Could you check a few things on this model? Use its own coordinates, in mm. A direction names the side the tool comes from. Give positions to 0.01 mm unless a question says otherwise; leave off trailing zeros. Loops run counter-clockwise (first coordinate to the right, second up) from the corner with the lowest first, then second, coordinate; pieces in that order, holes last. Notation, with made-up numbers: (88.25, 35.5) - (96.25, 35.5) arc R26 cw to (96.25, 59.5) - close; hole circle Ø1 at (37, 33). An arc over 180 degrees is marked (long way). Write each question's results on one line, items separated by ' | '. Start each with the question number.
(1) Suppose I cut it at B-B (y = 7.5). Please give me the cut outline in (x, z).
(2) Suppose I cut it at D-D (y = 4.75). Please give me the cut outline in (x, z), and give its area (3 significant figures).
(3) Suppose I cut it at C-C (x = -9.3). Please give me the cut outline in (y, z).
(4) For pin 1 (5 mm diameter, centred on x = -9.5, z = -17.5, fed in from +Y); pin 2 (8 mm diameter, centred on x = -13, z = -16.5, fed in from -Y); pin 3 (10 mm diameter, centred on x = -16.5, y = 16, fed in from -Z); pin 4 (3 mm diameter, centred on x = -4.5, z = -4.9, fed in from -Y), each with a flat end and sliding along its axis, tell me the tip position at first contact or that it passes through.
(5) Suppose I cut it at A-A (z = -4.9). Please give me the cut outline in (x, y).
(6) I need wall thicknesses on line 1 (X direction, y = 5.25, z = -30.1); line 2 (Z direction, x = -4.5, y = 3.75); line 3 (Z direction, x = -14.1, y = 4.75). Which ranges of each line are inside material? Lowest first, please.
(7) If we mould it in two halves opening along X, with no side actions, what happens to faces 4 (the face through (0, 7, -18)), 5 (the face through (-14.188, 3.944, -32.098)), 6 (the face through (-9.17, 3.21, -24.5))? For each: released by +X, released by -X, zero draft, split by the parting line, or undercut.
(8) On a 3-axis mill with a long thin cutter (end or side, diameter ignored), from which of +Z, -Z, +X, -X, +Y, -Y can I reach the whole of each face in a straight line? I mean faces 1 (the face through (-9.17, 3.298, -10.542)), 2 (the face through (-10.276, 13.423, -10.064)), 3 (the face through (-18.6, 7, -17)). Say none if no direction works.
Autodesk Inventor part; units mm, degrees
ref_plane "YZ Plane" through (0, 0, 0) normal (1, 0, 0) x (0, 1, 0)
ref_plane "XZ Plane" through (0, 0, 0) normal (0, 1, 0) x (-1, 0, 0)
ref_plane "XY Plane" through (0, 0, 0) normal (0, 0, 1) x (1, 0, 0)
sketch "Esquisse1" plane through (0, 0, 0) normal (0, 1, 0) x (-1, 0, 0)
  line L0 (0, 0) -> (18.6, 0)
  line L1 (18.6, 0) -> (18.6, -35)
  line L2 (18.6, -35) -> (0, -35)
  line L3 (0, -35) -> (0, 0)
  dimension "d0" = 18.6
  dimension "d1" = 35
extrude "Extrusion1" add sketch "Esquisse1" along normal blind 8
sketch "Esquisse2" plane through (0, 0, 0) normal (1, 0, 0) x (0, 0, -1)
  line L0 (35, 0) -> (0, 0)
  line L1 (25.2, 0) -> (9.8, 0)
  line L2 (22.4477, 5.9) -> (12.5523, 5.9)
  arc A0 (25.2, 0) -> (22.4477, 5.9) centre (17.5, 0) ccw
  arc A1 (12.5523, 5.9) -> (9.8, 0) centre (17.5, 0) ccw
  dimension "d5" = 5.9
extrude "Extrusion2" cut sketch "Esquisse2" against normal up to surface (18.6 mm away)
ref_plane "Plan de construction1" through (-18.6, 0, -4.9) normal (0, 0, 1) x (1, 0, 0)
ref_plane "Plan de construction2" through (0, 0, -30.1) normal (0, 0, -1) x (-1, 0, 0)
ref_plane "Plan de construction3" through (-14.1, 0, 0) normal (-1, 0, 0) x (0, 0, 1)
ref_plane "Plan de construction4" through (-4.5, 0, -35) normal (1, 0, 0) x (0, 0, -1)
hole "Perçage1" at (-4.5, 8, -30.1) direction (0, -1, 0) diameter 4 depth 8
hole "Perçage2" at (-14.1, 8, -30.1) direction (0, -1, 0) diameter 4 depth 8
hole "Perçage3" at (-4.5, 8, -4.9) direction (0, -1, 0) diameter 4 depth 8
hole "Perçage4" at (-14.1, 8, -4.9) direction (0, -1, 0) diameter 4 depth 8
sketch "Esquisse3" plane through (0, 8, 0) normal (0, 1, 0) x (1, 0, 0)
  circle A0 centre (-9.3, 17.5) radius 7.5
  point P0 (0, 0)
  dimension "d48" = 15
extrude "Extrusion3" add sketch "Esquisse3" along normal blind 11
hole "Perçage5" at (-9.3, 19, -17.5) direction (0, -1, 0) diameter 6.3 depth 10
properties part number "bagueSilentbloc"
Output values:
1) outline: (-18.6, -35) - (0, -35) - (0, 0) - (-18.6, 0) - close; hole circle Ø4 at (-14.1, -30.1); hole circle Ø4 at (-14.1, -4.9); hole circle Ø4 at (-4.5, -30.1); hole circle Ø4 at (-4.5, -4.9)
2) outline: (-18.6, -35) - (0, -35) - (0, -23.56) - (-18.6, -23.56) - close; (-18.6, -11.44) - (0, -11.44) - (0, 0) - (-18.6, 0) - close; hole circle Ø4 at (-14.1, -30.1); hole circle Ø4 at (-14.1, -4.9); hole circle Ø4 at (-4.5, -30.1); hole circle Ø4 at (-4.5, -4.9) | area: 375 mm2
3) outline: (0, -35) - (8, -35) - (8, -25) - (19, -25) - (19, -20.65) - (9, -20.65) - (9, -14.35) - (19, -14.35) - (19, -10) - (8, -10) - (8, 0) - (0, 0) - (0, -9.8) arc R7.7 cw to (5.9, -12.55) - (5.9, -22.45) arc R7.7 cw to (0, -25.2) - close
4) pin 1: y = 9 | pin 2: y = 5.86 | pin 3: z = -24.67 | pin 4: through
5) outline: (-18.6, 0) - (-16.1, 0) - (-16.1, 8) - (-18.6, 8) - close; (-12.1, 0) - (-6.5, 0) - (-6.5, 8) - (-12.1, 8) - close; (-2.5, 0) - (0, 0) - (0, 8) - (-2.5, 8) - close
6) line 1: -18.6 to -16.1, -12.1 to -6.5, -2.5 to 0 | line 2: -35 to -32.1, -28.1 to -24.23, -10.77 to -6.9, -2.9 to 0 | line 3: -35 to -32.1, -28.1 to -23.56, -11.44 to -6.9, -2.9 to 0
7) face 4: released by +X | face 5: undercut | face 6: zero draft
8) face 1: +X, -X, -Y | face 2: +Y | face 3: +Z, -Z, -X, +Y, -Y
